Here's how the part is built. I have some questions about the finished solid (model axes, mm). Face numbers are marked on the shaded views. A direction names the side the tool comes from. Give positions to 0.01 mm unless a question says otherwise; leave off trailing zeros. Loops run counter-clockwise (first coordinate to the right, second up) from the corner with the lowest first, then second, coordinate; pieces in that order, holes last. Notation, with made-up numbers: (46.25, -11) -> (84.25, -11) arc R20 cw to (84.25, 6) -> close; hole circle Ø6 at (50, 47.25). An arc over 180 degrees is marked (long way). Answer in a Markdown table with one row per item. Add a question column.
Item 1: If we section it at D-D (y = 30): Write out the boundary of the cut face in (x, z), then the cut area to 3 significant figures.
Item 2: If we section it at B-B (z = -48.5): Write out the boundary of the cut face in (x, y) (3 decimals).
Item 3: For P1, Ø5, axis at y = 6.5, z = -14.5, coming from the +X side; P2, Ø2, axis at x = 32.5, y = 25, coming from the +Z side; P3, Ø8, axis at x = 29.5, y = 7.5, coming from the +Z side, each with a flat end and sliding along its axis, tell me the tip position at first contact or that it passes through.
Item 4: We'd pull the mould along Z, two halves only. Please class the marked faces 4, 5 and 6: released by +Z, released by -Z, zero draft, split by the parting line, or undercut.
Item 5: If I drill on line 1 (X direction, y = 4, z = -2.5) (3 decimals); line 2 (Y direction, x = 11.5, z = -42.5); line 3 (Z direction, x = 70, y = 24), over which ranges is the centre line in solid material (lowest first)?
Item 6: Which directions (+Z, -Z, +X, -X, +Y, -Y) give clear straight access to the entire face, cutting with the end or side of a thin tool? Please do the marked faces 1, 2 and 3.
Item 7: If we section it at A-A (y = 5): Write out the boundary of the cut face in (x, z) (3 decimals).
Item 8: If we section it at C-C (x = 55): Write out the boundary of the cut face in (y, z).
```python
from build123d import *

# Parameters (mm, degrees)
ESQUISSE1_W                           = 95.25
ESQUISSE1_H                           = 57.15
BASE_EXTRUSION_DEPTH                  = 50.8
ENL_V_MAT_EXTRU_1_DEPTH               = 123.144688792
ESQUISSE3_W                           = 25.4
ESQUISSE3_H                           = 19.05
ESQUISSE3_W_2                         = 28.575
ESQUISSE3_H_2                         = 12.7
ENL_V_MAT_EXTRU_2_DEPTH               = 123.144688792
CHANFREIN1_SIZE                       = 19.05
ENL_V_MAT_EXTRU_3_DEPTH               = 123.144688792
DIAM_TRE_DU_PER_AGE_5_8_0_625_2_D     = 15.875
DIAM_TRE_DU_PER_AGE_5_8_0_625_2_DEPTH = 31.75
DIAM_TRE_DU_PER_AGE_5_8_0_625_2_TIP   = 4.769331164


with BuildPart() as part:
    # Esquisse1 → Base-Extrusion (new body)
    with BuildSketch(Plane(origin=(0, 0, 0), x_dir=(1, 0, 0), z_dir=(0, 1, 0))):
        with Locations((47.625, 28.575)):
            Rectangle(ESQUISSE1_W, ESQUISSE1_H)
    extrude(amount=BASE_EXTRUSION_DEPTH)

    # Esquisse2 → Enlèv. mat.-Extru.1 (cut, through all)
    with BuildSketch(Plane(origin=(95.25, 0, 0), x_dir=(0, 0, -1), z_dir=(1, 0, 0))):
        Polygon((44.45, 50.8), (0, 6.35), (0, 50.8), align=None)
    extrude(amount=-ENL_V_MAT_EXTRU_1_DEPTH, mode=Mode.SUBTRACT)

    # Esquisse3 → Enlèv. mat.-Extru.2 (cut, through all)
    with BuildSketch(Plane.XZ):
        with Locations((82.55, -9.525)):
            Rectangle(ESQUISSE3_W, ESQUISSE3_H)
        with Locations((39.6875, -6.35)):
            Rectangle(ESQUISSE3_W_2, ESQUISSE3_H_2)
    extrude(amount=-ENL_V_MAT_EXTRU_2_DEPTH, mode=Mode.SUBTRACT)

    # Chanfrein1
    chanfrein1_edges = [part.edges().sort_by_distance(p)[0] for p in [
        (95.25, 50.8, -50.8),
    ]]
    chamfer(chanfrein1_edges, length=CHANFREIN1_SIZE)

    # Esquisse4 → Enlèv. mat.-Extru.3 (cut, through all)
    with BuildSketch(Plane(origin=(0, 0, -57.15), x_dir=(-1, 0, 0), z_dir=(0, 0, -1))):
        Polygon((0, 50.8), (-47.625, 50.8), (-14.629432116, 31.75), (0, 31.75), align=None)
    extrude(amount=-ENL_V_MAT_EXTRU_3_DEPTH, mode=Mode.SUBTRACT)

    # Diamètre du perçage 5/8 (0.625)2
    with Locations(Plane(origin=(95.25, 0, 0), x_dir=(0, 0, -1), z_dir=(1, 0, 0))):
        with Locations((38.1, 15.875)):
            Hole(DIAM_TRE_DU_PER_AGE_5_8_0_625_2_D / 2, depth=DIAM_TRE_DU_PER_AGE_5_8_0_625_2_DEPTH)
            with Locations((0, 0, -(DIAM_TRE_DU_PER_AGE_5_8_0_625_2_DEPTH + DIAM_TRE_DU_PER_AGE_5_8_0_625_2_TIP / 2))):  # 118° drill point
                Cone(0, DIAM_TRE_DU_PER_AGE_5_8_0_625_2_D / 2, DIAM_TRE_DU_PER_AGE_5_8_0_625_2_TIP, mode=Mode.SUBTRACT)


solid = part.part
```
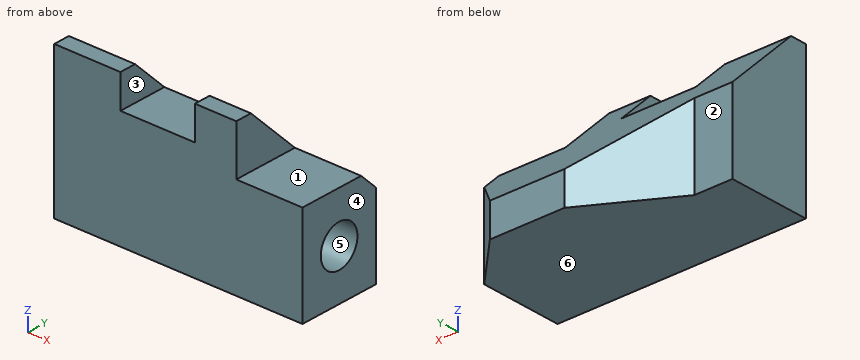
Recorded:
| question | item | result |
|---|---|---|
| 1 | outline | (0, -57.15) -> (95.25, -57.15) -> (95.25, -23.65) -> (0, -23.65) -> close |
| 1 | area | 3,190 mm^2 |
| 2 | outline | (0, 0) -> (95.25, 0) -> (95.25, 31.75) -> (76.2, 50.8) -> (47.625, 50.8) -> (14.629, 31.75) -> (0, 31.75) -> close |
| 3 | P1 | stops at x = 69.85 |
| 3 | P2 | stops at z = -17.65 |
| 3 | P3 | stops at z = -12.7 |
| 4 | face 4 | zero draft |
| 4 | face 5 | undercut |
| 4 | face 6 | released by -Z |
| 5 | line 1 | x = 0 to 25.4, 53.975 to 69.85 |
| 5 | line 2 | y = 0 to 31.75 |
| 5 | line 3 | z = -57.15 to -19.05 |
| 6 | face 1 | +Z, +X, +Y, -Y |
| 6 | face 2 | +Z, -Z, -X, +Y |
| 6 | face 3 | +Z, +Y, -Y |
| 7 | outline | (0, -57.15) -> (95.25, -57.15) -> (95.25, -19.05) -> (69.85, -19.05) -> (69.85, 0) -> (53.975, 0) -> (53.975, -12.7) -> (25.4, -12.7) -> (25.4, 0) -> (0, 0) -> close |
| 8 | outline | (0, -57.15) -> (50.8, -57.15) -> (50.8, -44.45) -> (6.35, 0) -> (0, 0) -> close |
